from build123d import *

# Parameters (mm, degrees)
SKETCH1_W           = 950
SKETCH1_H           = 460
BOSS_EXTRUDE2_DEPTH = 2
SKETCH3_R           = 3
CUT_EXTRUDE1_DEPTH  = 2
SKETCH5_W           = 450
SKETCH5_H           = 440
SKETCH5_R           = 3
BOSS_EXTRUDE3_DEPTH = 2


with BuildPart() as part:
    # Sketch1 → Boss-Extrude2 (new body)
    with BuildSketch(Plane(origin=(0, 0, 0), x_dir=(0, 0, -1), z_dir=(1, 0, 0))):
        Rectangle(SKETCH1_W, SKETCH1_H)
    extrude(amount=BOSS_EXTRUDE2_DEPTH)

    # Sketch3 → Cut-Extrude1 (cut)
    with BuildSketch(Plane(origin=(2, 0, 0), x_dir=(0, 0, -1), z_dir=(1, 0, 0))):
        with Locations((-400, 215)):
            Circle(SKETCH3_R)
        with Locations((-200, 215)):
            Circle(SKETCH3_R)
        with Locations((0, 215)):
            Circle(SKETCH3_R)
        with Locations((200, 215)):
            Circle(SKETCH3_R)
        with Locations((400, 215)):
            Circle(SKETCH3_R)
        with Locations(Location((400, -215, 0), (0, 0, 180))):
            Circle(SKETCH3_R)
        with Locations(Location((0, -215, 0), (0, 0, 180))):
            Circle(SKETCH3_R)
        with Locations(Location((200, -215, 0), (0, 0, 180))):
            Circle(SKETCH3_R)
        with Locations(Location((-200, -215, 0), (0, 0, 180))):
            Circle(SKETCH3_R)
        with Locations(Location((-400, -215, 0), (0, 0, 180))):
            Circle(SKETCH3_R)
    extrude(amount=-CUT_EXTRUDE1_DEPTH, mode=Mode.SUBTRACT)

    # Sketch5 → Boss-Extrude3 (add)
    with BuildSketch(Plane(origin=(2, 0, 0), x_dir=(0, 0, -1), z_dir=(1, 0, 0))):
        with Locations((250, 450)):
            Rectangle(SKETCH5_W, SKETCH5_H)
        with Locations((400, 655)):
            Circle(SKETCH5_R, mode=Mode.SUBTRACT)
        with Locations((200, 655)):
            Circle(SKETCH5_R, mode=Mode.SUBTRACT)
    extrude(amount=-BOSS_EXTRUDE3_DEPTH)


solid = part.part
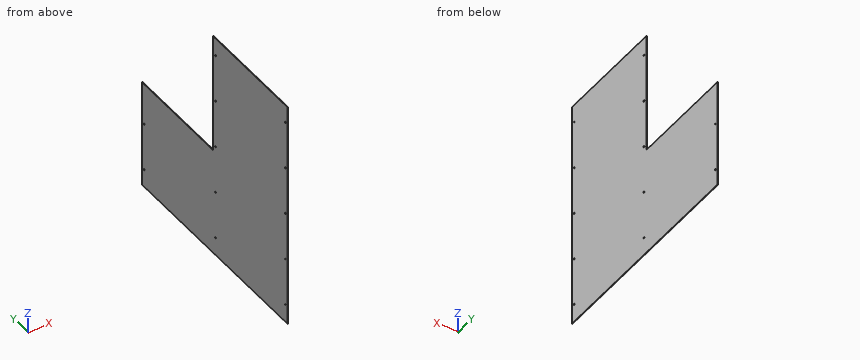
Geometry: final body of the model. Coordinates: model frame, mm. Give positions to 0.01 mm unless a question says otherwise; leave off trailing zeros. Write each loop counter-clockwise with the first axis right and the second up, starting at its lowest first coordinate (ties: lowest second). Pieces come first, ordered by that corner, then holes.
(1) Ray query, line 1 (Z direction, x = 1, y = 215); line 2 (Y direction, x = 0.5, z = 400); line 3 (Z direction, x = 1.35, y = 655). Return the intervals inside material, ascending.
(2) First-contact query: P1, Ø3.5, axis at y = 215, z = 0, coming from the -X side; P2, Ø1, axis at x = 1.5, y = 344, coming from the +Z side. Flat tips, straight axial feed; report the tip coordinate or a pass-through.
(3) Cut plane A-A, the plane x = 0.55. Give the number of separate pieces and of enclosed holes in the cut face, then the cut area to 3 significant figures.
(4) Cut plane B-B, the plane z = 109. Return loops of the section in (x, y).
(5) Cut plane C-C, the plane y = 494. Return loops of the section in (x, z).
Values follow:
1. line 1: z = -475 to -403, -397 to -203, -197 to -3, 3 to 197, 203 to 397, 403 to 475
1. line 2: y = -230 to -218, -212 to 212, 218 to 230
1. line 3: z = -475 to -403, -397 to -203, -197 to -25
2. P1: passes through
2. P2: stops at z = -25
3. separate pieces: 1
3. enclosed holes: 12
3. area: 635,000 mm2
4. outline: (0, -230) - (2, -230) - (2, 230) - (0, 230) - close
5. outline: (0, -475) - (2, -475) - (2, -25) - (0, -25) - close
